Can you work these out from the model? Positions are in its coordinate system, mm. Face numbers are marked on the shaded views. A direction names the side the tool comes from. Round coordinates to 2 decimals unless told otherwise and drop trailing zeros. Order: outer loops, then holes, each group sorted by start corner. A loop starts at its lowest first (then second) coordinate and runs counter-clockwise, first axis right, second up.
Q1. If we section it at A-A (x = 5.08): Please give me the cut outline in (y, z).
Q2. If we section it at C-C (z = 0): Please give me the cut outline in (x, y).
Q3. If we section it at D-D (x = 0): Please give me the cut outline in (y, z).
Q4. For the marked faces 1, 2 and 3, which set-ups out of +Z, -Z, +X, -X, +Y, -Y let a thin tool reach every point of the face, with its end or its side?
Q5. If I drill on line 1 (X direction, y = 0.7, z = 0); line 2 (Z direction, x = 4.75, y = -6.5); line 3 (X direction, y = -13.5, z = -19.5), over which ranges is the centre line in solid material (lowest first)?
Q6. Will these pins go through, and if not, where does the flat tip stop? P1, Ø6, axis at x = 6, y = -5.5, coming from the +Z side; P2, Ø5, axis at y = -1.5, z = -24.5, coming from the -X side; P3, Ø3, axis at y = -6.35, z = -13.34, coming from the -X side.
Q7. If we section it at B-B (y = -6.35): Please give me the cut outline in (x, z).
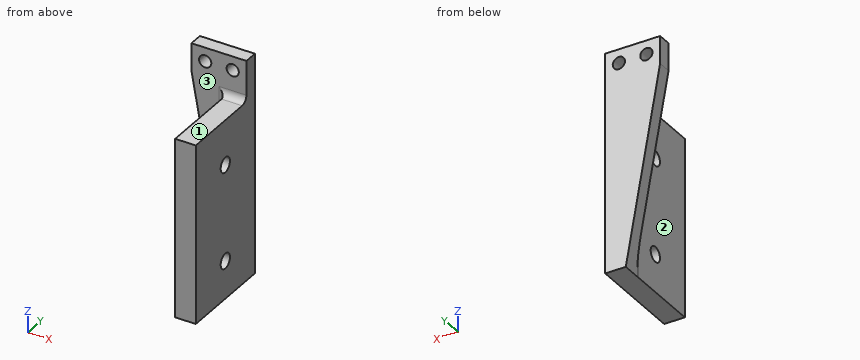
from build123d import *

# Parameters (mm, degrees)
SKETCH1_R           = 1.1303
BOSS_EXTRUDE1_DEPTH = 2.54
SKETCH2_W           = 3.81
SKETCH2_H           = 33.02
BOSS_EXTRUDE2_DEPTH = 15.24
FILLET1_R           = 1.27
SKETCH3_R           = 1.397
CUT_EXTRUDE1_DEPTH  = 12.7


with BuildPart() as part:
    # Sketch1 → Boss-Extrude1 (new body)
    with BuildSketch(Plane(origin=(0, 0, 0), x_dir=(1, 0, 0), z_dir=(0, 1, 0))):
        Polygon((-2.54, 2.54), (3.79857, 38.1), (7.60857, 38.1), (7.60857, 2.54), (7.60857, -2.54), (-2.54, -2.54), align=None)
        with Locations(Location((0, 0, 0), (0, 0, 270))):
            Circle(SKETCH1_R, mode=Mode.SUBTRACT)
        with Locations(Location((5.08, 0, 0), (0, 0, 270))):
            Circle(SKETCH1_R, mode=Mode.SUBTRACT)
    extrude(amount=BOSS_EXTRUDE1_DEPTH)

    # Sketch2 → Boss-Extrude2 (add)
    with BuildSketch(Plane.XZ):
        with Locations((5.70357, -21.59)):
            Rectangle(SKETCH2_W, SKETCH2_H)
    extrude(amount=BOSS_EXTRUDE2_DEPTH)

    # Fillet1
    fillet1_edges = [part.edges().sort_by_distance(p)[0] for p in [
        (5.70357, 0, -5.08),
        (3.79857, 0, -21.59),
    ]]
    fillet(fillet1_edges, radius=FILLET1_R)

    # Sketch3 → Cut-Extrude1 (cut)
    with BuildSketch(Plane(origin=(7.60857, 0, 0), x_dir=(0, 0, -1), z_dir=(1, 0, 0))):
        with Locations((13.335254, -6.35)):
            Circle(SKETCH3_R)
        with Locations((31.115254, -6.35)):
            Circle(SKETCH3_R)
    extrude(amount=-CUT_EXTRUDE1_DEPTH, mode=Mode.SUBTRACT)


solid = part.part
Solution:
1. outline: (-15.24, -38.1) - (2.54, -38.1) - (2.54, -1.13) - (0, -1.13) - (0, -3.81) arc R1.27 cw to (-1.27, -5.08) - (-15.24, -5.08) - close; (0, 1.13) - (2.54, 1.13) - (2.54, 2.54) - (0, 2.54) - close; hole circle Ø2.79 at (-6.35, -31.12); hole circle Ø2.79 at (-6.35, -13.34)
2. outline: (-2.54, 0) - (-1.13, 0) - (-1.13, 2.54) - (-2.54, 2.54) - close; (1.13, 0) - (3.95, 0) - (3.95, 2.54) - (1.13, 2.54) - close; (6.21, 0) - (7.61, 0) - (7.61, 2.54) - (6.21, 2.54) - close
3. outline: (0, -16.79) - (2.54, -16.79) - (2.54, -1.13) - (0, -1.13) - close; (0, 1.13) - (2.54, 1.13) - (2.54, 2.54) - (0, 2.54) - close
4. face 1: +Z, +X, -X, -Y
4. face 2: +Z, -Z, -X, -Y
4. face 3: +Z, -X, -Y
5. line 1: x = -2.54 to -1.13, 1.13 to 3.95, 6.21 to 7.61
5. line 2: z = -38.1 to -32.5, -29.73 to -14.72, -11.95 to -5.08
5. line 3: x = 3.8 to 7.61
6. P1: stops at z = -5.08
6. P2: stops at x = 1.02
6. P3: stops at x = 3.8
7. outline: (3.8, -38.1) - (7.61, -38.1) - (7.61, -32.51) - (3.8, -32.51) - close; (3.8, -29.72) - (7.61, -29.72) - (7.61, -14.73) - (3.8, -14.73) - close; (3.8, -11.94) - (7.61, -11.94) - (7.61, -5.08) - (3.8, -5.08) - close
